```python
from build123d import *

# Parameters (mm, degrees)
SKETCH_1_R          = 2
EXTRUDE_1_DEPTH     = 7.8
CUT_EXTRUDE_START   = 3.5
SKETCH_2_R          = 2
SKETCH_2_R_2        = 1.5
CUT_EXTRUDE_1_DEPTH = 0.5
SKETCH_3_R          = 0.71
CUT_EXTRUDE_2_DEPTH = 0.5
SKETCH_4_W          = 3.57211422
SKETCH_4_H          = 1.8
EXTRUDE_2_DEPTH     = 5.5
SKETCH_5_RX         = 1.78605711
SKETCH_5_RY         = 0.9
EXTRUDE_3_DEPTH     = 3.3


with BuildPart() as part:
    # 草图1 → 凸台-拉伸1 (new body)
    with BuildSketch(Plane.XY):
        Circle(SKETCH_1_R)
    extrude(amount=EXTRUDE_1_DEPTH)

    # 草图2 → 切除-拉伸1 (cut)
    with BuildSketch(Plane.XY.offset(CUT_EXTRUDE_START)):
        Circle(SKETCH_2_R)
        Circle(SKETCH_2_R_2, mode=Mode.SUBTRACT)
    extrude(amount=CUT_EXTRUDE_1_DEPTH, mode=Mode.SUBTRACT)

    # 草图3 → 切除-拉伸2 (cut)
    with BuildSketch(Plane.XY.offset(7.8)):
        Circle(SKETCH_3_R)
    extrude(amount=-CUT_EXTRUDE_2_DEPTH, mode=Mode.SUBTRACT)

    # 草图4 → 凸台-拉伸2 (add)
    with BuildSketch(Plane.XY):
        Rectangle(SKETCH_4_W, SKETCH_4_H)
    extrude(amount=-EXTRUDE_2_DEPTH)

    # 草图5 → 凸台-拉伸3 (add)
    with BuildSketch(Plane(origin=(0, 0, -5.5), x_dir=(-1, 0, 0), z_dir=(0, 0, -1))):
        with Locations((0, 0)):
            Ellipse(SKETCH_5_RX, SKETCH_5_RY)
    extrude(amount=EXTRUDE_3_DEPTH)


solid = part.part
```
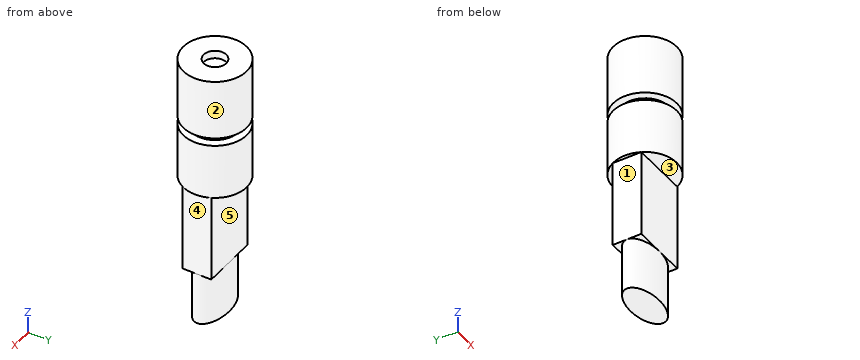
For this review, take the finished solid that the model builds, in its own axes (mm). Face numbers are marked on the shaded views. A direction names the side the tool comes from. Round coordinates to 2 decimals unless told otherwise and drop trailing zeros. Write each loop counter-clockwise with the first axis right and the second up, starting at its lowest first coordinate (ties: lowest second). Pieces come first, ordered by that corner, then holes.
1) Machinability: for the marked faces 1, 2, 3, 4 and 5, which of the approach directions +Z, -Z, +X, -X, +Y, -Y give a long, thin tool a straight path to every point of the face, cutting with its end or side? Answer none if there is none.
Answer below:
face 1: -Z, -X, +Y, -Y
face 2: +Z, -Z
face 3: -Z, +X, -X, -Y
face 4: -Z, +X, +Y, -Y
face 5: -Z, +X, -X, +Y
2) Insertion check: pin 1 Ø2 at (y, z) = (0, -2) entering from +X; pin 2 Ø2 at (y, z) = (0, -4) entering from -X; pin 3 Ø2 at (x, z) = (1.5, 0.5) entering from -Y. Each pin has a flat end and moves straight along its axis. Give the tip position at first contact, or say it passes through.
Answer below:
pin 1: stops at x = 1.79
pin 2: stops at x = -1.79
pin 3: stops at y = -1.94
3) Take a section at C-C on z = 3. Give the boundary of the cut face in (x, y).
Answer below:
outline: circle Ø4 at (0, 0)
4) Take a section at A-A on y = 1.2. Give the boundary of the cut face in (x, z), then the cut area to 3 significant figures.
Answer below:
outline: (-1.6, 0) - (1.6, 0) - (1.6, 3.5) - (0.9, 3.5) - (0.9, 4) - (1.6, 4) - (1.6, 7.8) - (-1.6, 7.8) - (-1.6, 4) - (-0.9, 4) - (-0.9, 3.5) - (-1.6, 3.5) - close
area: 24.3 mm2
5) Take a section at B-B on z = -2. Give the boundary of the cut face in (x, y).
Answer below:
outline: (-1.79, -0.9) - (1.79, -0.9) - (1.79, 0.9) - (-1.79, 0.9) - close
6) For line 1 along Z through (x, y) = (1.65, -0.2); line 2 along Y through (x, z) = (0, 7.55); line 3 along X through (y, z) = (0.65, -1.5), list the stretches that pass through material, from the lowest coordinate up.
Answer below:
line 1: z = -8.8 to 3.5, 4 to 7.8
line 2: y = -2 to -0.71, 0.71 to 2
line 3: x = -1.79 to 1.79
